Source: CAD feature listing. Evaluate the final solid. Frame: model axes, mm. A direction names the side the tool comes from. Coordinates: 2 decimals unless noted, no trailing zeros. Order: outer loops, then holes, each group sorted by start corner. A loop starts at its lowest first (then second) coordinate and runs counter-clockwise, first axis right, second up. Notation, with made-up numbers: (48, 3.25) -> (90, 3.25) arc R14 ccw to (90, 17.25) -> close; hole circle Ø2 at (38, 18.5). An arc over 180 degrees is marked (long way). Write each question's results on one line, items separated by ' | '. Start each with the question number.
from build123d import *

# Parameters (mm, degrees)
SKETCH1_W                                      = 50.8
SKETCH1_H                                      = 9.525
EXTRUDE1_DEPTH                                 = 10
SKETCH2_R                                      = 15.24
CUT_EXTRUDE1_DEPTH                             = 10.525
CBORE_FOR_6_SOCKET_HEAD_CAP_SCREW1_D           = 3.7973
CBORE_FOR_6_SOCKET_HEAD_CAP_SCREW1_CBORE_D     = 7.14502
CBORE_FOR_6_SOCKET_HEAD_CAP_SCREW1_CBORE_DEPTH = 3.5052


with BuildPart() as part:
    # Sketch1 → Extrude1 (new body)
    with BuildSketch(Plane(origin=(0, 0, 0), x_dir=(1, 0, 0), z_dir=(0, 1, 0))):
        with Locations((-25.4, 4.7625)):
            Rectangle(SKETCH1_W, SKETCH1_H)
    extrude(amount=EXTRUDE1_DEPTH)

    # Sketch2 → Cut-Extrude1 (cut, through all)
    with BuildSketch(Plane(origin=(0, 0, -9.525), x_dir=(-1, 0, 0), z_dir=(0, 0, -1))):
        with Locations((25.4, 20.24)):
            Circle(SKETCH2_R)
    extrude(amount=-CUT_EXTRUDE1_DEPTH, mode=Mode.SUBTRACT)

    # CBORE for #6 Socket Head Cap Screw1 (through all)
    with Locations(Plane(origin=(-43.18, 0, -4.7625), x_dir=(0, 0, -1), z_dir=(0, -1, 0))):
        with Locations((0, 0), (0.0635, 35.559943304)):
            CounterBoreHole(CBORE_FOR_6_SOCKET_HEAD_CAP_SCREW1_D / 2, CBORE_FOR_6_SOCKET_HEAD_CAP_SCREW1_CBORE_D / 2, CBORE_FOR_6_SOCKET_HEAD_CAP_SCREW1_CBORE_DEPTH)


solid = part.part
(1) Draft query along X for faces 1 (the cylindrical face through (-39.638, 1.728, -4.297)), 2 (the flat face through (0, 5, -5)), 3 (the flat face through (-5.6, 10, -5.9)). Return one class per face: released by +X, released by -X, zero draft, split by the parting line, or undercut.
(2) First-contact query: P1, Ø2, axis at x = -7.5, z = -5, coming from the -Y side; P2, Ø4.5, axis at x = -43.18, z = -4.76, coming from the -Y side; P3, Ø4, axis at x = -24.5, z = -4.5, coming from the +Y side. Flat tips, straight axial feed; report the tip coordinate or a pass-through.
(3) Section B-B on z = -4. Return the cut outline in (x, y), then the cut area to 3 significant figures.
(4) Section D-D on x = -7. Return the cut outline in (y, z) (3 decimals).
(5) Section A-A on x = -43.18. Return the cut outline in (y, z) (3 decimals), then the cut area to 3 significant figures.
(6) Section C-C on y = 2.5. Return the cut outline in (x, z) (1 decimal).
(7) Line query: L1, parallel to X at y = 2.75, z = -2; L2, parallel to X at y = 4.5, z = -5; L3, parallel to Y at x = -5.5, z = -6. Output: solid intervals per line, ascending.
(8) Reachability of faces 4 (the flat face through (-26, 4, 0)), 5 (the flat face through (-45, 3.505, -6)) from +Z, -Z, +X, -X, +Y, -Y: full face, straight path, thin tool, end or side. Return the list, or none.
Results list:
1) face 1: undercut | face 2: released by +X | face 3: zero draft
2) P1: passes through | P2: stops at y = 3.51 | P3: stops at y = 5.28
3) outline: (-50.8, 0) -> (-46.67, 0) -> (-46.67, 3.51) -> (-44.92, 3.51) -> (-44.92, 10) -> (-50.8, 10) -> close; (-41.44, 3.51) -> (-39.69, 3.51) -> (-39.69, 0) -> (-11.1, 0) -> (-11.1, 3.51) -> (-9.33, 3.51) -> (-9.33, 10) -> (-14.11, 10) arc R15.24 cw to (-36.69, 10) -> (-41.44, 10) -> close; (-5.91, 3.51) -> (-4.14, 3.51) -> (-4.14, 0) -> (0, 0) -> (0, 10) -> (-5.91, 10) -> close | area: 336 mm²
4) outline: (0, -9.525) -> (10, -9.525) -> (10, -6.621) -> (3.505, -6.621) -> (3.505, -8.344) -> (0, -8.344) -> close; (0, -1.308) -> (3.505, -1.308) -> (3.505, -3.031) -> (10, -3.031) -> (10, 0) -> (0, 0) -> close
5) outline: (0, -9.525) -> (10, -9.525) -> (10, -6.661) -> (3.505, -6.661) -> (3.505, -8.335) -> (0, -8.335) -> close; (0, -1.19) -> (3.505, -1.19) -> (3.505, -2.864) -> (10, -2.864) -> (10, 0) -> (0, 0) -> close | area: 45.5 mm²
6) outline: (-50.8, -9.5) -> (0, -9.5) -> (0, 0) -> (-50.8, 0) -> close; hole circle Ø7.1 at (-43.2, -4.8); hole circle Ø7.1 at (-7.6, -4.8)
7) L1: x = -50.8 to -45.45, -40.91 to -9.81, -5.43 to 0 | L2: x = -50.8 to -45.06, -41.3 to -9.51, -5.73 to 0 | L3: y = 3.51 to 10
8) face 4: +Z, +X, -X, +Y, -Y | face 5: -Y
